from build123d import *

# Parameters (mm, degrees)
CUT_EXTRUDE2_DEPTH = 53.77783625727755
SKETCH4_R          = 1.5999999999999994
CUT_EXTRUDE3_DEPTH = 46.594955861366955
SKETCH2_R          = 12.5
CUT_EXTRUDE4_DEPTH = 10


with BuildPart() as part:
    # Sketch1 → Revolve1 (revolve)
    with BuildSketch(Plane.XY, mode=Mode.PRIVATE) as revolve1_sk:
        Polygon((0.1, 0), (0.1, 24.900000000000002), (10.9, 24.900000000000002), (10.9, 36.50000000000001), (10.700000000000001, 36.50000000000001), (10.700000000000001, 25.1), (-0.1, 25.1), (-0.1, 0), align=None)
    revolve(revolve1_sk.sketch.rotate(Axis((0, 0, 0), (1, 0, 0)), 90), axis=Axis((0, 0, 0), (1, 0, 0)))

    # Sketch3 → Cut-Extrude2 (cut, through all)
    with BuildSketch(Plane.ZY.offset(0.1)):
        with BuildLine():
            Line((-10, 23.02194605153985), (-10, 35.10341863693621))
            ThreePointArc((-10, 35.10341863693621), (-36.50000000000001, 4.47e-15), (-10.000000000000007, -35.103418636936205))
            Line((-9.999999999999996, -35.10341863693621), (-9.999999999999996, -23.021946051539842))
            ThreePointArc((-9.999999999999691, -23.02194605153974), (-25.1, 3.07e-15), (-9.999999999999675, 23.021946051539746))
        make_face()
        with BuildLine():
            ThreePointArc((36.50000000000001, 0), (29.131168874592042, 21.991475621249254), (9.999999999999995, 35.10341863693621))
            Line((10, 35.10341863693621), (10, 23.021946051539338))
            ThreePointArc((10.000000000000362, 23.021946051539448), (20.98821097664126, 13.766081504916185), (25.1, 0))
            ThreePointArc((25.1, -6.15e-15), (20.98821097664126, -13.766081504916182), (10.000000000000357, -23.02194605153945))
            Line((9.999999999999996, -23.021946051539338), (9.999999999999996, -35.10341863693621))
            ThreePointArc((9.999999999999995, -35.10341863693621), (29.13116887459203, -21.991475621249272), (36.50000000000001, -8.94e-15))
        make_face()
    extrude(amount=-CUT_EXTRUDE2_DEPTH, mode=Mode.SUBTRACT)

    # Sketch4 → Cut-Extrude3 (cut, through all)
    with BuildSketch(Plane.ZY.offset(-10.700000000000001)):
        with Locations((0, 33)):
            Circle(SKETCH4_R)
        with Locations((0, -33)):
            Circle(SKETCH4_R)
    extrude(amount=-CUT_EXTRUDE3_DEPTH, mode=Mode.SUBTRACT)

    # Sketch2 → Cut-Extrude4 (cut)
    with BuildSketch(Plane.ZY.offset(0.1)):
        Circle(SKETCH2_R)
    extrude(amount=-CUT_EXTRUDE4_DEPTH, mode=Mode.SUBTRACT)


solid = part.part
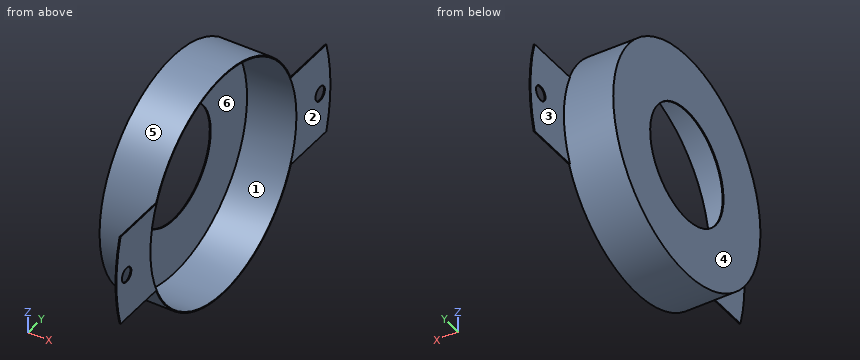
Here's how the part is built. I have some questions about the finished solid (model axes, mm). Face numbers are marked on the shaded views. A direction names the side the tool comes from. Give positions to 0.01 mm unless a question says otherwise; leave off trailing zeros. Write each loop counter-clockwise with the first axis right and the second up, starting at its lowest first coordinate (ties: lowest second). Pieces come first, ordered by that corner, then holes. Notation, with made-up numbers: (82, 3) -> (94, 3) arc R15 ccw to (94, 14) -> close; hole circle Ø6 at (-25.5, 9.25). An arc over 180 degrees is marked (long way). Use one line per item in the form item = value. Start each with the question number.
1. Imagine slicing it at D-D on z = -16. List the corners of the cut face in (x, y) for me, plus the area to 3 significant figures.
2. Thinking about a two-plate mould opening in X: for the marked faces 1, 2 and 3, which applies, +X half, -X half, draft (parallel to the pull), parting line (faces both ways), or undercut?
3. Imagine slicing it at C-C on x = 1.5. List the corners of the cut face in (y, z) for me.
4. Imagine slicing it at A-A on y = 33. List the corners of the cut face in (x, z) for me, plus the area to 3 significant figures.
5. If I drill on L1, parallel to Y at x = 10.85, z = 0; L2, parallel to Y at x = 8, z = 0; L3, parallel to Y at x = 10.25, z = -4, over which ranges is the centre line in solid material (lowest first)?
6. Imagine slicing it at B-B on z = 0. List the corners of the cut face in (x, y) for me, plus the area to 3 significant figures.
7. Will these pins go through, and if not, where does the flat tip stop? pin 1 Ø15 at (y, z) = (0, 0) entering from -X; pin 2 Ø1.5 at (x, z) = (4, -7) entering from -Y; pin 3 Ø2 at (x, z) = (6.5, 13) entering from -Y; pin 4 Ø1 at (x, z) = (7.5, 4.5) entering from -Y.
8. On a 3-axis mill with a long thin cutter (end or side, diameter ignored), from which of +Z, -Z, +X, -X, +Y, -Y can I reach the whole of each face in a straight line? I mean the marked faces 4, 5 and 6. Say none if no direction works.
Entries:
q1.outline = (-0.1, -19.34) -> (10.9, -19.34) -> (10.9, -19.08) -> (0.1, -19.08) -> (0.1, 19.08) -> (10.9, 19.08) -> (10.9, 19.34) -> (-0.1, 19.34) -> close
q1.area = 13.4 mm²
q2.face_1 = draft
q2.face_2 = +X half
q2.face_3 = -X half
q3.outline = circle Ø50.2 at (0, 0); hole circle Ø49.8 at (0, 0)
q4.outline = (10.7, -10) -> (10.9, -10) -> (10.9, -1.6) -> (10.7, -1.6) -> close; (10.7, 1.6) -> (10.9, 1.6) -> (10.9, 10) -> (10.7, 10) -> close
q4.area = 3.36 mm²
q5.L1 = -36.5 to -34.6, -31.4 to -24.9, 24.9 to 31.4, 34.6 to 36.5
q5.L2 = -25.1 to -24.9, 24.9 to 25.1
q5.L3 = -24.78 to -24.58, 24.58 to 24.78
q6.outline = (-0.1, -25.1) -> (10.7, -25.1) -> (10.7, -31.4) -> (10.9, -31.4) -> (10.9, -24.9) -> (0.1, -24.9) -> (0.1, -12.5) -> (-0.1, -12.5) -> close; (-0.1, 12.5) -> (0.1, 12.5) -> (0.1, 24.9) -> (10.9, 24.9) -> (10.9, 31.4) -> (10.7, 31.4) -> (10.7, 25.1) -> (-0.1, 25.1) -> close; (10.7, -36.5) -> (10.9, -36.5) -> (10.9, -34.6) -> (10.7, -34.6) -> close; (10.7, 34.6) -> (10.9, 34.6) -> (10.9, 36.5) -> (10.7, 36.5) -> close
q6.area = 12.6 mm²
q7.pin_1 = through
q7.pin_2 = -24.31
q7.pin_3 = -22.05
q7.pin_4 = -24.78
q8.face_4 = +Z, -Z, -X, +Y, -Y
q8.face_5 = -X
q8.face_6 = +X
